Autodesk Inventor part; units mm, degrees
ref_plane "YZ Plane" through (0, 0, 0) normal (1, 0, 0) x (0, 1, 0)
ref_plane "XZ Plane" through (0, 0, 0) normal (0, 1, 0) x (-1, 0, 0)
ref_plane "XY Plane" through (0, 0, 0) normal (0, 0, 1) x (1, 0, 0)
sketch "Sketch1" plane through (0, 0, 0) normal (1, 0, 0) x (0, 1, 0)
  line L0 (-25, 15) -> (25, 15)
  line L1 (25, 15) -> (25, -15)
  line L2 (25, -15) -> (-25, -15)
  line L3 (-25, -15) -> (-25, 15)
  line L4 (-25, 15) -> (25, -15) construction
  line L5 (25, 15) -> (-25, -15) construction
  line L6 (-15, -9) -> (15, -9) construction
  line L7 (15, -9) -> (15, 9) construction
  line L8 (15, 9) -> (-15, 9) construction
  line L9 (-15, 9) -> (-15, -9) construction
  line L10 (-15, -9) -> (15, 9) construction
  line L11 (15, -9) -> (-15, 9) construction
  circle A0 centre (15, -9) radius 1.65
  circle A1 centre (15, 9) radius 1.65
  circle A2 centre (-15, 9) radius 1.65
  circle A3 centre (-15, -9) radius 1.65
  point P0 (0, 0)
  dimension "d0" = 50
  dimension "d1" = 30
  dimension "d4" = 30
  dimension "d5" = 3.3
extrude "Extrusion1" add sketch "Sketch1" against normal blind 6
sketch "Sketch2" plane through (0, 0, 0) normal (1, 0, 0) x (0, 0, -1)
  line L0 (15, -25) -> (15, 25)
  line L1 (15, 25) -> (-15, 25)
  line L2 (-15, 25) -> (-15, -25)
  line L3 (-15, -25) -> (15, -25)
  circle A0 centre (9, -15) radius 1.65
  circle A1 centre (-9, -15) radius 1.65
  circle A2 centre (-9, 15) radius 1.65
  circle A3 centre (9, 15) radius 1.65
  line L4 (-15, -7.5) -> (15, -7.5)
  line L5 (15, -7.5) -> (15, 7.5)
  line L6 (15, 7.5) -> (-15, 7.5)
  line L7 (-15, 7.5) -> (-15, -7.5)
  line L8 (-15, -7.5) -> (15, 7.5) construction
  line L9 (15, -7.5) -> (-15, 7.5) construction
  point P0 (0, 0)
  point P1 (-15, 7.5)
  point P2 (-15, -7.5)
  dimension "d6" = 15
extrude "Extrusion2" add sketch "Sketch2" along normal blind 9 contours L4 L2 L6 L0
sketch "Sketch3" plane through (9, 0, 0) normal (1, 0, 0) x (0, 0, -1)
  line L0 (-15, 7.5) -> (-15, -7.5)
  line L1 (-15, -7.5) -> (15, -7.5)
  line L2 (15, -7.5) -> (15, 7.5)
  line L3 (15, 7.5) -> (-15, 7.5)
  line L4 (-15, -7.5) -> (15, -7.5)
  line L5 (15, -7.5) -> (15, 17.5)
  line L6 (15, 17.5) -> (-15, 17.5)
  line L7 (-15, 17.5) -> (-15, -7.5)
  point P0 (0, 0)
  dimension "d9" = 25
extrude "Extrusion3" add sketch "Sketch3" along normal blind 5
sketch "Sketch4" plane through (14, 0, 0) normal (1, 0, 0) x (0, 0, -1)
  line L0 (-15, 7.5) -> (15, 7.5)
  line L1 (15, 7.5) -> (-15, 7.5)
  line L2 (-15, -7.5) -> (15, -7.5)
  line L3 (15, -7.5) -> (15, 17.5)
  line L4 (15, 17.5) -> (-15, 17.5)
  line L5 (-15, 17.5) -> (-15, -7.5)
  point P0 (0, 0)
  point P1 (15, 7.5)
  point P2 (-15, 7.5)
extrude "Extrusion4" add sketch "Sketch4" along normal blind 2.5 contours L0 L3 L2 L5
sketch "Sketch5" plane through (16.5, 0, 0) normal (1, 0, 0) x (0, 0, -1)
  line L0 (-15, 7.5) -> (15, 7.5)
  line L1 (15, 7.5) -> (15, 17.5)
  line L2 (15, 17.5) -> (-15, 17.5)
  line L3 (-15, 17.5) -> (-15, 7.5)
  line L4 (15, -7.5) -> (15, 7.5)
  line L5 (15, 7.5) -> (-15, 7.5)
  line L6 (-15, 7.5) -> (-15, -7.5)
  line L7 (-15, -7.5) -> (15, -7.5)
  point P0 (0, 0)
extrude "Extrusion5" add sketch "Sketch5" along normal blind 5
chamfer "Chamfer1" distance 3 angle 45 2 edges at (14, 17.5, 0) (16.5, 17.5, 0)
sketch "Sketch6" plane through (14, 7.5, 15) normal (0, 1, 0) x (1, 0, 0)
  line L0 (0, 0) -> (0, 30)
  line L1 (0, 0) -> (2.5, 0)
  line L2 (2.5, 30) -> (2.5, 0)
  line L3 (0, 30) -> (2.5, 30)
  point P0 (-14, 15)
extrude "Extrusion6" cut sketch "Sketch6" against normal blind 6
chamfer "Chamfer2" distance 3 angle 45 4 edges at (-3, 25, 15) (-3, 25, -15) (-3, -25, -15) (-3, -25, 15)
fillet "Fillet1" radius 2 3 edges at (0, 7.5, 0) (0, -7.5, 0) (21.5, -7.5, 0)
properties part number "SEGURO" material "Steel, Mild, Welded"
The model under review builds one solid part; all positions refer to its coordinate system, in mm. A direction names the side the tool comes from. Coordinates: 2 decimals unless noted, no trailing zeros. Order: outer loops, then holes, each group sorted by start corner. A loop starts at its lowest first (then second) coordinate and runs counter-clockwise, first axis right, second up. Notation, with made-up numbers: (23, 66.5) -> (71, 66.5) arc R23 ccw to (71, 95.5) -> close; hole circle Ø7 at (-15, 49.5). An arc over 180 degrees is marked (long way). Answer in a Markdown table with one row per item.
(1) Consider section C-C (y = -15). Write out the cut boundary in (x, z).
Answers:
| item | result |
|---|---|
| outline | (-6, -15) -> (0, -15) -> (0, -10.65) -> (-6, -10.65) -> close; (-6, -7.35) -> (0, -7.35) -> (0, 7.35) -> (-6, 7.35) -> close; (-6, 10.65) -> (0, 10.65) -> (0, 15) -> (-6, 15) -> close |
(2) Consider section D-D (z = 4.5). Write out the cut boundary in (x, y).
Answers:
| item | result |
|---|---|
| outline | (-6, -25) -> (0, -25) -> (0, -9.5) arc R2 cw to (2, -7.5) -> (19.5, -7.5) arc R2 ccw to (21.5, -5.5) -> (21.5, 17.5) -> (19.5, 17.5) -> (16.5, 14.5) -> (16.5, 1.5) -> (14, 1.5) -> (14, 14.5) -> (11, 17.5) -> (9, 17.5) -> (9, 7.5) -> (2, 7.5) arc R2 cw to (0, 9.5) -> (0, 25) -> (-6, 25) -> close |
(3) Consider section A-A (z = -9). Write out the cut boundary in (x, y).
Answers:
| item | result |
|---|---|
| outline | (-6, -25) -> (0, -25) -> (0, -16.65) -> (-6, -16.65) -> close; (-6, -13.35) -> (0, -13.35) -> (0, -9.5) arc R2 cw to (2, -7.5) -> (19.5, -7.5) arc R2 ccw to (21.5, -5.5) -> (21.5, 17.5) -> (19.5, 17.5) -> (16.5, 14.5) -> (16.5, 1.5) -> (14, 1.5) -> (14, 14.5) -> (11, 17.5) -> (9, 17.5) -> (9, 7.5) -> (2, 7.5) arc R2 cw to (0, 9.5) -> (0, 13.35) -> (-6, 13.35) -> close; (-6, 16.65) -> (0, 16.65) -> (0, 25) -> (-6, 25) -> close |
(4) The part is to be moulded in two halves that separate along Z. For faces 4 (the cylindrical face through (0.57, -8.1, -0.21)), 5 (the flat face through (-3, 24, 13)), 6 (the cylindrical face through (-2.958, -13.476, 8.368)), 7 (the flat face through (8, 0, -15)), say which applies: +Z half, -Z half, draft (parallel to the pull), parting line (faces both ways), or undercut.
Answers:
| item | result |
|---|---|
| face 4 | draft |
| face 5 | +Z half |
| face 6 | undercut |
| face 7 | -Z half |
(5) Insertion check: pin 1 (5.5 mm diameter, centred on y = -15, z = -9, fed in from -X); pin 2 (14 mm diameter, centred on x = 12, z = 5, fed in from -Y); pin 3 (5 mm diameter, centred on x = 14, z = -10, fed in from +Y); pin 4 (0.8 mm diameter, centred on x = 15.5, z = -2, fed in from +Y). Each pin has a flat end and moves straight along its axis. Give the tip position at first contact, or say it passes through.
Answers:
| item | result |
|---|---|
| pin 1 | x = -6 |
| pin 2 | y = -7.5 |
| pin 3 | y = 17 |
| pin 4 | y = 1.5 |
(6) Wall thickness on line 1 along X through (y, z) = (10.5, 10.5); line 2 along Z through (x, y) = (-4.5, 15); line 3 along X through (y, z) = (9, -2): over which ranges is each line inside the solid? List them lowest first.
Answers:
| item | result |
|---|---|
| line 1 | -6 to 0, 9 to 14, 16.5 to 21.5 |
| line 2 | -15 to -10.65, -7.35 to 7.35, 10.65 to 15 |
| line 3 | -6 to 0.06, 9 to 14, 16.5 to 21.5 |
(7) Machinability: for faces 1 (the flat face through (20, 17.5, 0)), 2 (the flat face through (15, 1.5, 0)), 3 (the flat face through (0, -17, 0)), which of the approach directions +Z, -Z, +X, -X, +Y, -Y give a long, thin tool a straight path to every point of the face, cutting with its end or side? Answer none if there is none.
Answers:
| item | result |
|---|---|
| face 1 | +Z, -Z, +X, +Y |
| face 2 | +Z, -Z, +Y |
| face 3 | +Z, -Z, +X, -Y |
(8) Consider section B-B (y = 5). Write out the cut boundary in (x, z).
Answers:
| item | result |
|---|---|
| outline | (-6, -15) -> (14, -15) -> (14, 15) -> (-6, 15) -> close; (16.5, -15) -> (21.5, -15) -> (21.5, 15) -> (16.5, 15) -> close |
